```python
from build123d import *

# Parameters (mm, degrees)
F1_DEPTH = 6
F3_DEPTH = 6.001
F4_R     = 1


with BuildPart() as f1:
    # F0 (on Top) → F1 (new body)
    with BuildSketch(Plane.XY):
        with BuildLine():
            ThreePointArc((-4.7055641516, 7.671875), (0, -9), (4.7055641516, 7.671875))
            ThreePointArc((4.7055641516, 7.671875), (0, 15.25), (-4.7055641516, 7.671875))
        make_face()
        with BuildLine():
            ThreePointArc((1.0429029122, 6.921875), (0, -7), (-1.0429029122, 6.921875))
            ThreePointArc((-1.0429029122, 6.921875), (0, 13.25), (1.0429029122, 6.921875))
        make_face(mode=Mode.SUBTRACT)
    extrude(amount=F1_DEPTH)

    # F2 (on face) → F3 (cut, through all)
    with BuildSketch(Plane.XY.offset(6)):
        with BuildLine():
            ThreePointArc((0.5, -6.9821200219), (0, -7), (-0.5, -6.9821200219))
            Line((-0.5, -6.9821200219), (-2.2234871513, -8.7210151294))
            ThreePointArc((-2.2234871513, -8.7210151294), (-1.1204605827, -8.9299814156), (0, -9))
            ThreePointArc((0, -9), (1.1204605827, -8.9299814156), (2.2234871513, -8.7210151294))
            Line((2.2234871513, -8.7210151294), (0.5, -6.9821200219))
        make_face()
    extrude(amount=-F3_DEPTH, mode=Mode.SUBTRACT)

    # F4
    f4_edges = [f1.edges().sort_by_distance(p)[0] for p in [
        (-1.042903, 6.921875, 3),
        (4.705564, 7.671875, 3),
        (2.223487, -8.721015, 3),
        (-2.223487, -8.721015, 3),
        (-4.705564, 7.671875, 3),
        (1.042903, 6.921875, 3),
    ]]
    fillet(f4_edges, radius=F4_R)


solid = f1.part
```
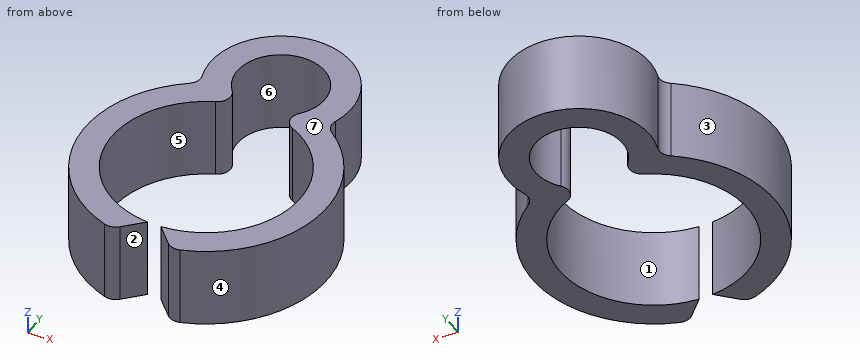
The model under review builds one solid part; all positions refer to its coordinate system, in mm. Face numbers are marked on the shaded views. A direction names the side the tool comes from. Give positions to 0.01 mm unless a question says otherwise; leave off trailing zeros. Write each loop counter-clockwise with the first axis right and the second up, starting at its lowest first coordinate (ties: lowest second). Pieces come first, ordered by that corner, then holes. Notation, with made-up numbers: (89.5, 7.25) - (144.5, 7.25) arc R21 ccw to (144.5, 41.25) - close; hole circle Ø5 at (17, 47). An arc over 180 degrees is marked (long way). Answer in a Markdown table with one row per item. Add a question column.
1. We need section A-A on y = 10. Write out the cut boundary in (x, z), then the cut area to 3 significant figures.
2. Wall thickness on line 1 along X through (y, z) = (10, 4); line 2 along Y through (x, z) = (-1.75, 1); line 3 along Y through (x, z) = (-3, 4.75): over which ranges is each line inside the solid? List them lowest first. Write a range as [from, to].
3. Tool access review of the marked faces 1, 2 and 3: name each direction out of +Z, -Z, +X, -X, +Y, -Y from which nothing blocks a thin tool from reaching the whole face with its end or side.
4. We need section B-B on x = -0.75. Write out the cut boundary in (y, z), then the cut area to 3 significant figures.
5. Draft analysis for pull direction Y (two halves, no side actions). For the marked faces 4, 5, 6 and 7, state which applies: +Y half, -Y half, draft (parallel to the pull), parting line (faces both ways), or undercut.
6. Insertion check: P1, Ø6, axis at x = -2.5, y = -4.5, coming from the -Z side; P2, Ø2, axis at y = -4, z = 3.5, coming from the -X side; P3, Ø1.5, axis at y = 5, z = 2, coming from the -X side. Each pin has a flat end and moves straight along its axis. Give the tip position at first contact, or say it passes through.
Ans:
| question | item | result |
|---|---|---|
| 1 | outline | (-5.25, 0) - (-3.25, 0) - (-3.25, 6) - (-5.25, 6) - close; (3.25, 0) - (5.25, 0) - (5.25, 6) - (3.25, 6) - close |
| 1 | area | 24.0 mm^2 |
| 2 | line 1 | x = [-5.25, -3.25], [3.25, 5.25] |
| 2 | line 2 | y = [-8.24, -6.78], [12.74, 14.95] |
| 2 | line 3 | y = [-8.49, -6.32], [6.32, 8.75], [11.25, 14.31] |
| 3 | face 1 | +Z, -Z |
| 3 | face 2 | +Z, -Z, -Y |
| 3 | face 3 | +Z, -Z, -X |
| 4 | outline | (-7.23, 0) - (-6.96, 0) - (-6.96, 6) - (-7.23, 6) - close; (13.16, 0) - (15.2, 0) - (15.2, 6) - (13.16, 6) - close |
| 4 | area | 13.9 mm^2 |
| 5 | face 4 | parting line |
| 5 | face 5 | undercut |
| 5 | face 6 | undercut |
| 5 | face 7 | draft |
| 6 | P1 | stops at z = 0 |
| 6 | P2 | stops at x = -8.49 |
| 6 | P3 | stops at x = -7.93 |
